Could you check a few things on this model? Use its own coordinates, in mm. Face numbers are marked on the shaded views. Round coordinates to 2 decimals unless told otherwise and drop trailing zeros. Order: outer loops, then holes, each group sorted by start corner. A loop starts at its lowest first (then second) coordinate and runs counter-clockwise, first axis right, second up. Notation, with made-up numbers: (24.25, 43) - (44.25, 43) arc R21 ccw to (44.25, 72) - close; hole circle Ø5 at (85, -39). An arc over 180 degrees is marked (long way). Use one line per item in the form item = value.
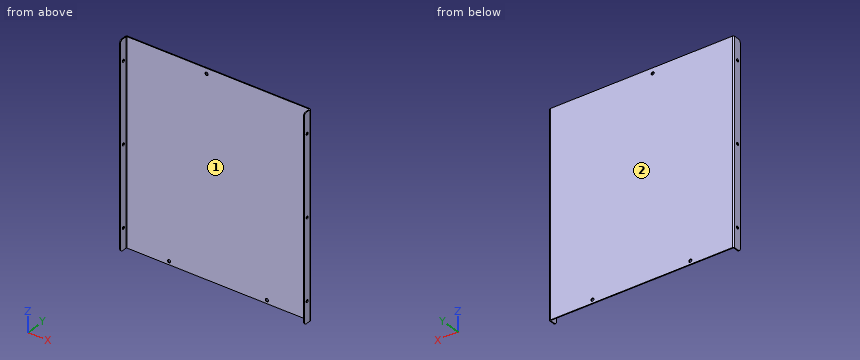
from build123d import *

# Parameters (mm, degrees)
SKETCH1_W                    = 211.5
SKETCH1_H                    = 227.5
BASE_FLANGE1_DEPTH           = 1
EDGE_FLANGE1_STRIP_W         = 5
EDGE_FLANGE1_STRIP_H         = 1
EDGE_FLANGE1_STRIP_CUT_DEPTH = 227.5
EDGE_FLANGE1_DEPTH           = 227.5
EDGE_FLANGE2_STRIP_W         = 5
EDGE_FLANGE2_STRIP_H         = 1
EDGE_FLANGE2_STRIP_CUT_DEPTH = 227.5
EDGE_FLANGE2_DEPTH           = 227.5
SKETCH13_R                   = 1.6
CUT_EXTRUDE1_DEPTH           = 241.356636064
FILLET1_R                    = 3
SKETCH14_R                   = 1.75
CUT_EXTRUDE2_DEPTH           = 156.634588058
SKETCH15_R                   = 1.75
CUT_EXTRUDE3_DEPTH           = 156.634588058


# Sheet-metal steps are written as plain solids
with BuildPart() as part:
    # Sketch1 → Base-Flange1 (new body)
    with BuildSketch(Plane(origin=(0, 0, 0), x_dir=(1, 0, 0), z_dir=(0, 1, 0))):
        Rectangle(SKETCH1_W, SKETCH1_H)
    extrude(amount=-BASE_FLANGE1_DEPTH)

    # Edge-Flange1 strip (across the edge) → Edge-Flange1 strip cut (cut)
    with BuildSketch(Plane(origin=(105.75, -1, -113.75), x_dir=(-1, 0, 0), z_dir=(0, 0, 1))):
        with Locations((-1, -0.5)):
            Rectangle(EDGE_FLANGE1_STRIP_W, EDGE_FLANGE1_STRIP_H)
    extrude(amount=EDGE_FLANGE1_STRIP_CUT_DEPTH, mode=Mode.SUBTRACT)

    # Edge-Flange1 section (across the edge) → Edge-Flange1 (add)
    with BuildSketch(Plane(origin=(105.75, -1, -113.75), x_dir=(-1, 0, 0), z_dir=(0, 0, 1))):
        with BuildLine():
            Line((0, 0.5), (0, 9))
            Line((0, 9), (1, 9))
            Line((1, 9), (1, 0.5))
            ThreePointArc((1, 0.5), (1.146446609, 0.146446609), (1.5, 0))
            Line((1.5, 0), (1.5, -1))
            ThreePointArc((1.5, -1), (0.439339828, -0.560660172), (0, 0.5))
        make_face()
    extrude(amount=EDGE_FLANGE1_DEPTH)

    # Edge-Flange2 strip (across the edge) → Edge-Flange2 strip cut (cut)
    with BuildSketch(Plane(origin=(-105.75, -1, 113.75), x_dir=(1, 0, 0), z_dir=(0, 0, -1))):
        with Locations((-1, -0.5)):
            Rectangle(EDGE_FLANGE2_STRIP_W, EDGE_FLANGE2_STRIP_H)
    extrude(amount=EDGE_FLANGE2_STRIP_CUT_DEPTH, mode=Mode.SUBTRACT)

    # Edge-Flange2 section (across the edge) → Edge-Flange2 (add)
    with BuildSketch(Plane(origin=(-105.75, -1, 113.75), x_dir=(1, 0, 0), z_dir=(0, 0, -1))):
        with BuildLine():
            Line((0, 0.5), (0, 9))
            Line((0, 9), (1, 9))
            Line((1, 9), (1, 0.5))
            ThreePointArc((1, 0.5), (1.146446609, 0.146446609), (1.5, 0))
            Line((1.5, 0), (1.5, -1))
            ThreePointArc((1.5, -1), (0.439339828, -0.560660172), (0, 0.5))
        make_face()
    extrude(amount=EDGE_FLANGE2_DEPTH)

    # Sketch13 → Cut-Extrude1 (cut, through all)
    with BuildSketch(Plane.ZY.offset(105.75)):
        with Locations(Location((0, -5.75, 0), (0, 0, 270))):
            Circle(SKETCH13_R)
        with Locations(Location((90, -5.75, 0), (0, 0, 270))):
            Circle(SKETCH13_R)
        with Locations(Location((-90, -5.75, 0), (0, 0, 270))):
            Circle(SKETCH13_R)
    extrude(amount=-CUT_EXTRUDE1_DEPTH, mode=Mode.SUBTRACT)

    # Fillet1
    fillet1_edges = [part.edges().sort_by_distance(p)[0] for p in [
        (105.25, -10, -113.75),
        (105.25, -10, 113.75),
        (-105.25, -10, 113.75),
        (-105.25, -10, -113.75),
    ]]
    fillet(fillet1_edges, radius=FILLET1_R)

    # Sketch14 → Cut-Extrude2 (cut, through all)
    with BuildSketch(Plane(origin=(0, 0, 0), x_dir=(1, 0, 0), z_dir=(0, 1, 0))):
        with Locations(Location((-56, 109.95, 0), (0, 0, 270))):
            Circle(SKETCH14_R)
        with Locations(Location((56, 109.95, 0), (0, 0, 270))):
            Circle(SKETCH14_R)
    extrude(amount=-CUT_EXTRUDE2_DEPTH, mode=Mode.SUBTRACT)

    # Sketch15 → Cut-Extrude3 (cut, through all)
    with BuildSketch(Plane(origin=(0, 0, 0), x_dir=(1, 0, 0), z_dir=(0, 1, 0))):
        with Locations(Location((-13, -107.75, 0), (0, 0, 270))):
            Circle(SKETCH15_R)
    extrude(amount=-CUT_EXTRUDE3_DEPTH, mode=Mode.SUBTRACT)


solid = part.part
Item 1: Imagine slicing it at A-A on z = -42. Please give me the cut outline in (x, y), plus the area to 3 significant figures.
Found:
outline = (-105.75, -10) - (-104.75, -10) - (-104.75, -1.5) arc R0.5 cw to (-104.25, -1) - (104.25, -1) arc R0.5 cw to (104.75, -1.5) - (104.75, -10) - (105.75, -10) - (105.75, -1.5) arc R1.5 ccw to (104.25, 0) - (-104.25, 0) arc R1.5 ccw to (-105.75, -1.5) - close
area = 229 mm2
Item 2: Imagine slicing it at B-B on x = -5. Please give me the cut outline in (y, z).
Found:
outline = (-1, -113.75) - (0, -113.75) - (0, 113.75) - (-1, 113.75) - close
Item 3: If we mould it in two halves opening along X, with no side actions, what happens to the marked faces 1 and 2? For each: released by +X, released by -X, zero draft, split by the parting line, or undercut.
Found:
face_1 = undercut
face_2 = zero draft
Item 4: Will this pin go through, and if not, where does the flat tip stop? P1, Ø4.5, axis at x = -13, z = 107.75, coming from the -Y side.
Found:
P1 = -1
Item 5: I need wall thicknesses on L1, parallel to Z at x = -105.05, y = -5.75; L2, parallel to X at y = -3.5, z = -49.5; L3, parallel to X at y = -0.6, z = -109.95. Which ranges of each line are inside material? Lowest first, please.
Found:
L1 = -113.75 to -91.6, -88.4 to -1.6, 1.6 to 88.4, 91.6 to 113.75
L2 = -105.75 to -104.75, 104.75 to 105.75
L3 = -105.45 to -57.75, -54.25 to 54.25, 57.75 to 105.45
